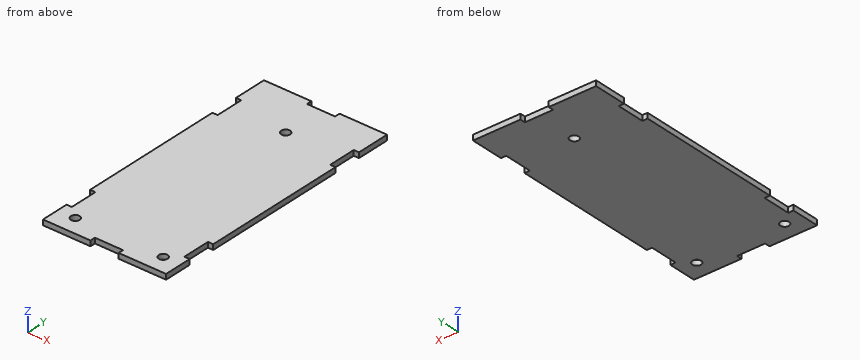
Autodesk Inventor part; units mm, degrees
ref_plane "YZ Plane" through (0, 0, 0) normal (1, 0, 0) x (0, 1, 0)
ref_plane "XZ Plane" through (0, 0, 0) normal (0, 1, 0) x (-1, 0, 0)
ref_plane "XY Plane" through (0, 0, 0) normal (0, 0, 1) x (1, 0, 0)
sketch "Sketch1" plane through (0, 0, 0) normal (0, 0, 1) x (1, 0, 0)
  line L0 (0, 0) -> (70, 0)
  line L1 (70, 0) -> (70, 150)
  line L2 (0, 131) -> (3, 131)
  line L3 (3, 131) -> (3, 115)
  line L4 (3, 115) -> (0, 115)
  line L5 (0, 115) -> (0, 131)
  line L6 (0, 32) -> (3, 32)
  line L7 (3, 32) -> (3, 16)
  line L8 (3, 16) -> (0, 16)
  line L9 (0, 16) -> (0, 32)
  line L10 (70, 131) -> (67, 131)
  line L11 (67, 131) -> (67, 115)
  line L12 (67, 115) -> (70, 115)
  line L13 (70, 115) -> (70, 131)
  line L14 (70, 32) -> (67, 32)
  line L15 (67, 32) -> (67, 16)
  line L16 (67, 16) -> (70, 16)
  line L17 (70, 16) -> (70, 32)
  line L18 (43, 150) -> (43, 147)
  line L19 (43, 147) -> (27, 147)
  line L20 (27, 147) -> (27, 150)
  line L21 (70, 150) -> (43, 150)
  line L22 (27, 150) -> (0, 150)
  line L23 (0, 150) -> (0, 131)
  line L24 (0, 115) -> (0, 0)
  line L25 (43, 0) -> (27, 0)
  line L26 (27, 0) -> (27, 3)
  line L27 (27, 3) -> (43, 3)
  line L28 (43, 3) -> (43, 0)
  point P0 (1.5, 16)
  point P1 (70, 123)
  point P2 (67, 123)
  dimension "d1" = 70
  dimension "d2" = 16
  dimension "d3" = 16
  dimension "d4" = 16
  dimension "d9" = 16
  dimension "d12" = 19
  dimension "d13" = 150
  dimension "d15" = 3
  dimension "d16" = 3
  dimension "d17" = 3
extrude "Plate1" add sketch "Sketch1" along normal blind 3 contours L24 L8 L7 L6 L4 L3 L2 L23 L22 L20 L19 L18 L21 L1 L10 L11 L12 L14 L15 L16 L0 L28 L27 L26
sketch "Sketch2" plane through (0, 0, 0) normal (0, 0, -1) x (-1, 0, 0)
  circle A0 centre (-35, 123) radius 2.5
  circle A1 centre (-60, 10) radius 2.5
  circle A2 centre (-10, 10) radius 2.5
  line L0 (-43, 147) -> (-27, 147)
  line L1 (-67, 131) -> (-67, 115)
  line L2 (-3, 131) -> (-3, 115)
  line L3 (0, 16) -> (-3, 16)
  line L4 (0, 0) -> (-27, 0)
  line L5 (0, 16) -> (0, 0)
  line L6 (-70, 0) -> (-70, 16)
  point P0 (-1.5, 16)
  point P1 (0, 8)
  dimension "d18" = 24
  dimension "d19" = 32
  dimension "d20" = 32
  dimension "d21" = 5
  dimension "d23" = 5
  dimension "d24" = 10
  dimension "d25" = 10
  dimension "d26" = 10
extrude "Extrusion1" cut sketch "Sketch2" against normal through all
equation "\"d14\" = Thickness"
equation "\"BendRadius\" = Thickness"
equation "\"BendReliefWidth\" = Thickness"
equation "\"BendReliefDepth\" = 0.5 * Thickness"
equation "\"CornerReliefSize\" = 4 * Thickness"
equation "\"MinimumRemnant\" = 2 * Thickness"
equation "\"TransitionRadius\" = BendRadius"
equation "\"JacobiRadiusSize\" = BendRadius"
equation "\"GapSize\" = Thickness"
properties part number "bottom plate" material "Hardboard"
CAD build for the part. Positions are in the model's coordinates, mm. Coordinates: 2 decimals unless noted, no trailing zeros. Order: outer loops, then holes, each group sorted by start corner. A loop starts at its lowest first (then second) coordinate and runs counter-clockwise, first axis right, second up.
(1) Saw through at B-B, the plane z = 0.55. Count the separate pieces of the cut face and the enclosed holes in it, and give its area (3 significant figures).
Solution:
separate pieces: 1
enclosed holes: 3
area: 10,200 mm2
(2) Saw through at C-C, the plane y = 10. Write the cut outline in (x, z).
Solution:
outline: (0, 0) - (7.5, 0) - (7.5, 3) - (0, 3) - close; (12.5, 0) - (57.5, 0) - (57.5, 3) - (12.5, 3) - close; (62.5, 0) - (70, 0) - (70, 3) - (62.5, 3) - close
(3) Saw through at D-D, the plane x = 60. Write the cut outline in (y, z).
Solution:
outline: (0, 0) - (7.5, 0) - (7.5, 3) - (0, 3) - close; (12.5, 0) - (150, 0) - (150, 3) - (12.5, 3) - close
(4) Saw through at A-A, the plane x = 35. Write the cut outline in (y, z), and give its area (3 significant figures).
Solution:
outline: (3, 0) - (120.5, 0) - (120.5, 3) - (3, 3) - close; (125.5, 0) - (147, 0) - (147, 3) - (125.5, 3) - close
area: 417 mm2
(5) Drill centre lines: L1, parallel to Y at x = 35, z = 1.3; L2, parallel to Y at x = 10, z = 2.35; L3, parallel to X at y = 9, z = 1.3. Where is each one in solid material? Low to high.
Solution:
L1: y = 3 to 120.5, 125.5 to 147
L2: y = 0 to 7.5, 12.5 to 150
L3: x = 0 to 7.71, 12.29 to 57.71, 62.29 to 70
(6) Pin check, flat tips, straight feed: pin 1 Ø4 at (x, y) = (35, 123) entering from -Z; pin 2 Ø1 at (y, z) = (30, 2.5) entering from +X. Stop position of each tip, or through.
Solution:
pin 1: passes through
pin 2: stops at x = 67
